```python
from build123d import *

# Parameters (mm, degrees)
EXTRUDE_1_DEPTH     = 7.5
SKETCH_4_R          = 20.03
SKETCH_4_R_2        = 9
CUT_EXTRUDE_1_DEPTH = 0.9375
CUT_EXTRUDE_1_DRAFT = -60
CHAMFER_2_SIZE      = 0.666666667


with BuildPart() as part:
    # 草图3 → 凸台-拉伸1 (new body)
    with BuildSketch(Plane(origin=(0, 0, 0), x_dir=(0, 0, -1), z_dir=(1, 0, 0))):
        Polygon((9, 5.196152423), (0, 10.392304845), (-9, 5.196152423), (-9, -5.196152423), (0, -10.392304845), (9, -5.196152423), align=None)
    extrude(amount=EXTRUDE_1_DEPTH)


with BuildPart() as cut_extrude_1_tool:
    # 草图4 → 切除-拉伸1 (with draft: the straight prism first)
    with BuildSketch(Plane.ZY):
        Circle(SKETCH_4_R)
        Circle(SKETCH_4_R_2, mode=Mode.SUBTRACT)
    extrude(amount=-CUT_EXTRUDE_1_DEPTH)
    # 切除-拉伸1: the draft: its side faces are tilted about the plane it starts from
    cut_extrude_1_sides = [cut_extrude_1_tool.faces().sort_by_distance(p)[0] for p in [
        (0.46875, 0, -20.03),
        (0.46875, 0, -9),
    ]]
    draft(cut_extrude_1_sides, Plane.ZY, CUT_EXTRUDE_1_DRAFT)


with BuildPart() as part_1:
    add(part.part)

    # 切除-拉伸1: cut by cut_extrude_1_tool
    add(cut_extrude_1_tool.part, mode=Mode.SUBTRACT)

    # 草图5 → 旋转1 (revolve)
    with BuildSketch(Plane.XY, mode=Mode.PRIVATE) as revolve_1_sk:
        with BuildLine():
            Line((8.35, 6), (47.5, 6))
            Line((47.5, 6), (47.5, 0))
            Line((47.5, 0), (7.5, 0))
            Line((7.5, 0), (7.5, 6.85))
            ThreePointArc((7.5, 6.85), (7.748959236, 6.248959236), (8.35, 6))
        make_face()
    revolve(revolve_1_sk.sketch.rotate(Axis((7.5, 0, 0), (1, 0, 0)), 90), axis=Axis((7.5, 0, 0), (1, 0, 0)))

    # 倒角2
    chamfer_2_edges = [part_1.edges().sort_by_distance(p)[0] for p in [
        (47.5, 0, -6),
    ]]
    chamfer(chamfer_2_edges, length=CHAMFER_2_SIZE)

    # 草图7 → 切除-旋转1 (revolve, cut)
    with BuildSketch(Plane.XY, mode=Mode.PRIVATE) as cut_revolve_1_sk:
        Polygon((7.5, 8.215), (6.9, 8.815), (6.9, 20.03), (7.5, 20.03), align=None)
    revolve(cut_revolve_1_sk.sketch.rotate(Axis((0, 0, 0), (1, 0, 0)), 90), axis=Axis((0, 0, 0), (1, 0, 0)), mode=Mode.SUBTRACT)


solid = part_1.part
```
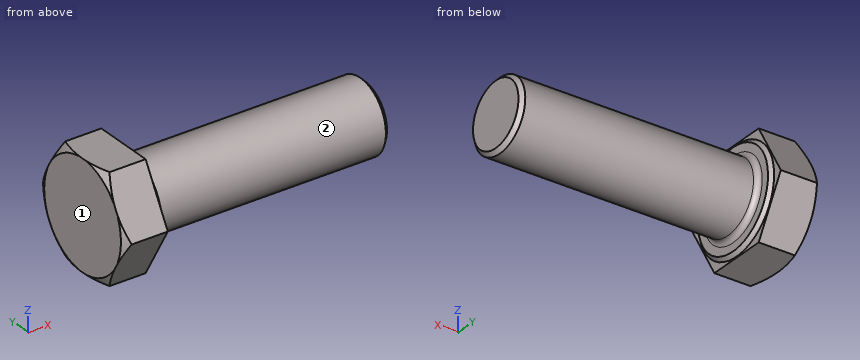
Source: CAD feature listing. Evaluate the final solid. Frame: model axes, mm. Face numbers are marked on the shaded views. A direction names the side the tool comes from. Coordinates: 2 decimals unless noted, no trailing zeros. Write each loop counter-clockwise with the first axis right and the second up, starting at its lowest first coordinate (ties: lowest second). Pieces come first, ordered by that corner, then holes. Notation, with made-up numbers: (28.25, 75) -> (76.25, 75) arc R15 ccw to (76.25, 103) -> close; hole circle Ø2 at (87.25, 86.5). An arc over 180 degrees is marked (long way). Return JSON: item names as keys, results as strings. Group by question number.
1) Ray query, line 1 along X through (y, z) = (-5.25, 6); line 2 along Y through (x, z) = (8.5, 0); line 3 along Y through (x, z) = (5, -5). Return the intervals inside material, ascending.
2) Contact query for flat-ended pins moving along their axis: P1, Ø3, axis at x = 21, z = 4.5, coming from the -Y side; P2, Ø6, axis at x = 42, z = -3.5, coming from the +Y side; P3, Ø2, axis at x = 6, z = -1.5, coming from the -Y side. Output: stop coordinate, or through.
3) Set-up query: the marked faces 1 and 2. Return all of +Z, -Z, +X, -X, +Y, -Y with unobstructed straight access to the full face (end or side cutting, diameter ignored); none if empty.
4) Section query A-A, the plane x = 39. Return loops of the section in (y, z), plus the area to 3 significant figures.
From the geometry:
{
 "1": {"line 1": "0 to 7.5", "line 2": "-6 to 6", "line 3": "-7.51 to 7.51"},
 "2": {"P1": "y = -5.2", "P2": "y = 5.98", "P3": "y = -10.1"},
 "3": {"face 1": "+Z, -Z, -X, +Y, -Y", "face 2": "+X"},
 "4": {"outline": "circle Ø12 at (0, 0)", "area": "113 mm²"}
}
